```python
from build123d import *

# Parameters (mm, degrees)
SCHIZZO1_R                   = 17.75
SCHIZZO1_R_2                 = 16.25
ESTRUSIONE_ESTRUSIONE1_DEPTH = 170
TAGLIO_ESTRUSIONE1_DEPTH     = 170
TAGLIO_ESTRUSIONE2_START     = -60
SCHIZZO4_R                   = 41.734641341
TAGLIO_ESTRUSIONE2_DEPTH     = 112.843315381
SCHIZZO5_R                   = 17.75
SCHIZZO6_R                   = 22.75
RACCORDO1_R                  = 1


with BuildPart() as part:
    # Schizzo1 → Estrusione-Estrusione1 (new body)
    with BuildSketch(Plane.XY):
        Circle(SCHIZZO1_R)
        Circle(SCHIZZO1_R_2, mode=Mode.SUBTRACT)
    extrude(amount=ESTRUSIONE_ESTRUSIONE1_DEPTH)

    # Schizzo2 → Taglio-Estrusione1 (cut)
    with BuildSketch(Plane(origin=(0, 0, 0), x_dir=(1, 0, 0), z_dir=(0, 1, 0))):
        with BuildLine():
            Line((-17.5, -25), (-17.5, -7.5))
            Line((-17.5, -7.5), (17.5, -7.5))
            Line((17.5, -7.5), (17.5, -25))
            ThreePointArc((17.5, -25), (0, -42.5), (-17.5, -25))
        make_face()
    extrude(amount=-TAGLIO_ESTRUSIONE1_DEPTH, mode=Mode.SUBTRACT)

    # Schizzo4 → Taglio-Estrusione2 (cut, through all)
    with BuildSketch(Plane(origin=(0, 0, 0), x_dir=(-1, 0, 0), z_dir=(0, 0, -1)).offset(TAGLIO_ESTRUSIONE2_START)):
        Circle(SCHIZZO4_R)
    extrude(amount=-TAGLIO_ESTRUSIONE2_DEPTH, mode=Mode.SUBTRACT)

    # Schizzo5 → Loft2 section 0
    with BuildSketch(Plane.XY.offset(60)):
        Circle(SCHIZZO5_R)
    # Schizzo6 → Loft2 section 1
    with BuildSketch(Plane.XY.offset(65)):
        Circle(SCHIZZO6_R)
    loft()

    # Schizzo9 → Taglia-Rivoluzione1 (revolve, cut)
    with BuildSketch(Plane(origin=(0, 0, 0), x_dir=(1, 0, 0), z_dir=(0, 1, 0)), mode=Mode.PRIVATE) as taglia_rivoluzione1_sk:
        Polygon((0, -53.809990156), (0, -67.47386211), (23.102541766, -67.47386211), (9.438669813, -53.809990156), align=None)
    revolve(taglia_rivoluzione1_sk.sketch.rotate(Axis((0, 0, 53.809990156), (0, 0, 1)), 180), axis=Axis((0, 0, 53.809990156), (0, 0, 1)), mode=Mode.SUBTRACT)

    # Raccordo1
    # the kernel refuses this fillet: 1 mm, written as the material it adds along each edge
    with BuildSketch(Plane(origin=(13.75, 0, 7.5), x_dir=(0, -1, 0), z_dir=(1, 0, 0))) as raccordo1_piece_1_section:
        with BuildLine():
            CenterArc((RACCORDO1_R, -RACCORDO1_R), RACCORDO1_R, 90, 90)
            Line((0, -RACCORDO1_R), (0, 0))
            Line((0, 0), (RACCORDO1_R, 0))
        make_face()
    raccordo1_piece_1 = extrude(amount=3.75, mode=Mode.PRIVATE)
    raccordo1_piece_1 = raccordo1_piece_1 - Plane(origin=(0, 0, 7.5), x_dir=(1, 0, 0), z_dir=(0, 0, -1)) * Cylinder(16.25, 12, mode=Mode.PRIVATE)
    add(raccordo1_piece_1)
    with BuildSketch(Plane(origin=(-17.5, 0, 7.5), x_dir=(0, -1, 0), z_dir=(1, 0, 0))) as raccordo1_piece_2_section:
        with BuildLine():
            CenterArc((RACCORDO1_R, -RACCORDO1_R), RACCORDO1_R, 90, 90)
            Line((0, -RACCORDO1_R), (0, 0))
            Line((0, 0), (RACCORDO1_R, 0))
        make_face()
    raccordo1_piece_2 = extrude(amount=3.75, mode=Mode.PRIVATE)
    raccordo1_piece_2 = raccordo1_piece_2 - Plane(origin=(0, 0, 7.5), x_dir=(1, 0, 0), z_dir=(0, 0, -1)) * Cylinder(16.25, 12, mode=Mode.PRIVATE)
    add(raccordo1_piece_2)
    with BuildSketch(Plane(origin=(0, 0, 60), x_dir=(1, 0, 0), z_dir=(0, 1, 0))) as raccordo1_piece_3:
        with BuildLine():
            CenterArc((17.75 + RACCORDO1_R, RACCORDO1_R * 0.414213562373), RACCORDO1_R, 180, 45)
            Line((17.75 + RACCORDO1_R * 0.292893218813, -RACCORDO1_R * 0.292893218813), (17.75, 0))
            Line((17.75, 0), (17.75, RACCORDO1_R * 0.414213562373))
        make_face()
    revolve(axis=Axis((0, 0, 60), (0, 0, -1)))
    # the kernel refuses this fillet: 1 mm, written as the material it takes off along each edge
    with BuildSketch(Plane(origin=(0, 0, 60), x_dir=(-1, 0, 0), z_dir=(0, -1, 0))) as raccordo1_2_piece_1:
        with BuildLine():
            CenterArc((17.231963548, -0.18907033), RACCORDO1_R, 169.101465323, 55.898534677)
            Line((16.524856767, -0.896177111), (15.628679656, 0))
            Line((15.628679656, 0), (16.25, 0))
        make_face()
    revolve(axis=Axis((0, 0, 60), (0, 0, -1)), mode=Mode.SUBTRACT)


solid = part.part
```
Geometry: final body of the model. Coordinates: model frame, mm. A direction names the side the tool comes from. Give positions to 0.01 mm unless a question says otherwise; leave off trailing zeros. Loops run counter-clockwise (first coordinate to the right, second up) from the corner with the lowest first, then second, coordinate; pieces in that order, holes last. Notation, with made-up numbers: (73, -14) -> (115, -14) arc R20 ccw to (115, 8) -> close; hole circle Ø7 at (44, 57). An arc over 180 degrees is marked (long way). Return JSON: item names as keys, results as strings.
Item 1: Mould query, pull axis Y, two halves, no side actions, for faces 1 (the flat face through (16, -5, 0)), 2 (the cylindrical face through (-2.3, 17.6, 29.4)), 3 (the conical face through (13.272, 10.176, 61.095)). Classes: released by +Y, released by -Y, zero draft, split by the parting line, or undercut.
Filled in:
{"face 1": "zero draft", "face 2": "split by the parting line", "face 3": "undercut"}
Item 2: Section B-B, the plane z = 48.5. Output: boundary loops of the cut face in (x, y).
Filled in:
{"outline": "circle Ø35.5 at (0, 0); hole circle Ø32.5 at (0, 0)"}
Item 3: Section A-A, the plane x = 0. Output: boundary loops of the cut face in (y, z), plus the area to 3 significant figures.
Filled in:
{"outline": "(-22.75, 65) -> (-18.04, 60.29) arc R1 cw to (-17.75, 59.59) -> (-17.75, 42.5) -> (-16.25, 42.5) -> (-16.25, 60) arc R1 ccw to (-16.52, 60.9) -> (-20.63, 65) -> close; (-17.75, 0) -> (-16.25, 0) -> (-16.25, 7.5) -> (-17.75, 7.5) -> close; (16.25, 0) -> (17.75, 0) -> (17.75, 59.59) arc R1 cw to (18.04, 60.29) -> (22.75, 65) -> (20.63, 65) -> (16.52, 60.9) arc R1 ccw to (16.25, 60) -> close", "area": "148 mm^2"}
Item 4: Line query: line 1 (X direction, y = 0, z = 46); line 2 (Y direction, x = 0, z = 20.5); line 3 (Y direction, x = -9, z = 41). Output: solid intervals per line, ascending.
Filled in:
{"line 1": "-17.75 to -16.25, 16.25 to 17.75", "line 2": "16.25 to 17.75", "line 3": "-15.3 to -13.53, 13.53 to 15.3"}
Item 5: Section C-C, the plane y = -10. Count the separate pieces of the cut face and the enclosed holes in it, plus the area to 3 significant figures.
Filled in:
{"separate pieces": "4", "enclosed holes": "0", "area": "142 mm^2"}
Item 6: Pin query (flat end, axial travel): P1, Ø8.5, axis at x = -1.5, y = -13.5, coming from the +Z side; P2, Ø2, axis at x = -4.5, z = 10.5, coming from the -Y side; P3, Ø1.5, axis at x = -4.5, z = 30, coming from the +Y side. Return the tip coordinate at first contact, or that it passes through.
Filled in:
{"P1": "z = 62.2", "P2": "y = 15.29", "P3": "y = 17.35"}
Item 7: Access query for faces 4 (the conical face through (-3.975, -17.901, 60.587)), 5 (the cylindrical face through (6.11, -15.43, 41.4)). Directions: +Z, -Z, +X, -X, +Y, -Y. A direction counts if a zero-diameter tool reaches every point of the face in a straight line with its end or side. Return the directions, or none.
Filled in:
{"face 4": "-Z", "face 5": "-Y"}
